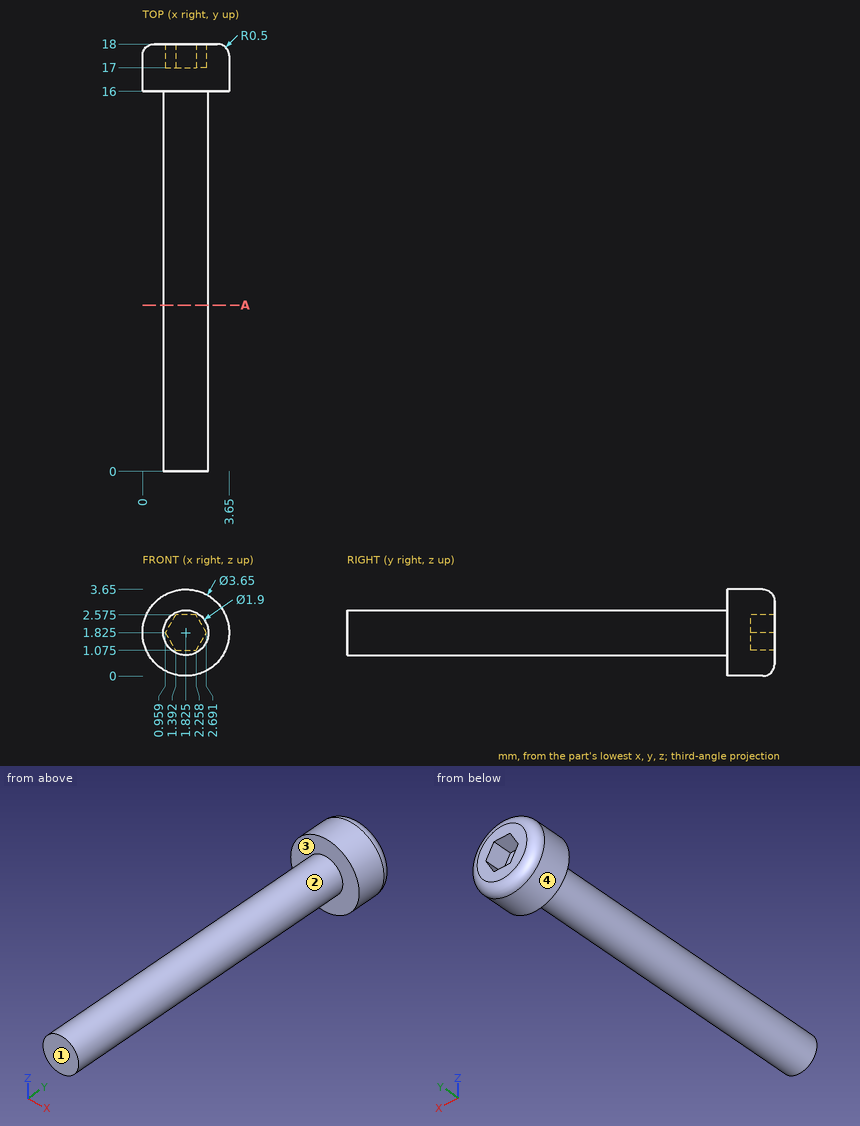
Study the drawing (mm; zero at the part's minimum x, y, z) and answer. A direction names the side the tool comes from. Round coordinates to 2 decimals unless told otherwise and drop trailing zeros. Write each loop counter-clockwise with the first axis right and the second up, starting at its lowest first coordinate (ties: lowest second). Pieces come first, ordered by that corner, then holes. Notation, with made-up numbers: (-12.75, 71.25) - (23.25, 71.25) arc R34 ccw to (23.25, 107.25) - close; hole circle Ø2 at (32.5, 70). An arc over 180 degrees is marked (long way). Use a Markdown table: item, result. Add a question column.
1. For a pull along Y with two mould halves and no side action, classify the marked faces 1 and 2 as +Y half, -Y half, draft (parallel to the pull), parting line (faces both ways), or undercut.
2. The part is cut by section A-A (y = 7). Write down the section's boundary in (x, z) (3 decimals), and give its area (3 significant figures).
3. Flat-ended cylindrical pins translate along their axes: P1, Ø1, axis at y = 8.5, z = 1, coming from the -X side; P2, Ø1, axis at x = 2, y = 11.5, coming from the +Z side (3 decimals); P3, Ø0.8, axis at x = 2, z = 2, coming from the +Y side. Find the tip coordinate at first contact, or state that the pin passes through.
4. A tool of negligible diameter and unlimited length cuts with its end or side. For the marked faces 3 and 4, from which of +Z, -Z, +X, -X, +Y, -Y can it reach the whole face along a straight path? Write none if from no direction.
5. Consider line 1 (Y direction, x = 2.5, z = 2.85); line 2 (Y direction, x = 2.2, z = 1.6); line 3 (X direction, y = 15.5, z = 1.8). Determine where each line is inside the solid, lowest interval first.
Reported:
| question | item | result |
|---|---|---|
| 1 | face 1 | -Y half |
| 1 | face 2 | draft |
| 2 | outline | circle Ø1.9 at (1.825, 1.825) |
| 2 | area | 2.84 mm^2 |
| 3 | P1 | x = 0.93 |
| 3 | P2 | z = 2.775 |
| 3 | P3 | y = 17 |
| 4 | face 3 | -Y |
| 4 | face 4 | +Y, -Y |
| 5 | line 1 | 16 to 18 |
| 5 | line 2 | 0 to 17 |
| 5 | line 3 | 0.88 to 2.77 |
